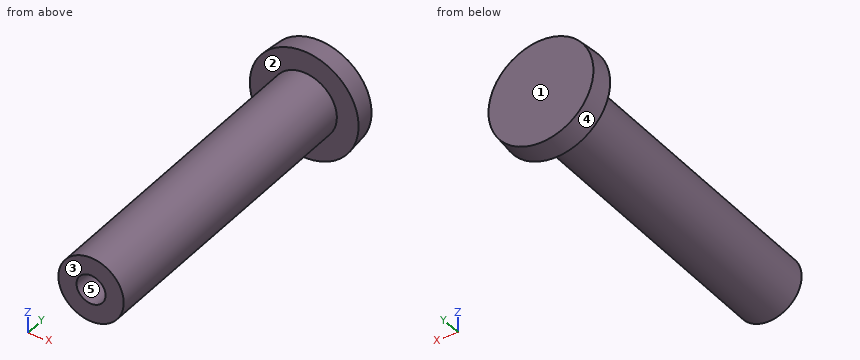
from build123d import *

# Parameters (mm, degrees)
SKETCH1_R           = 2.25
BOSS_EXTRUDE1_DEPTH = 21.5
SKETCH2_R           = 3.75
BOSS_EXTRUDE2_DEPTH = 1.5
BOSS_EXTRUDE2_TAPER = 5
SKETCH3_R           = 1
CUT_EXTRUDE1_DEPTH  = 6
CUT_EXTRUDE1_DRAFT  = -1


with BuildPart() as part:
    # Sketch1 → Boss-Extrude1 (new body)
    with BuildSketch(Plane(origin=(0, 0, 0), x_dir=(1, 0, 0), z_dir=(0, 1, 0))):
        with Locations(Location((0, 0, 0), (0, 0, 270))):
            Circle(SKETCH1_R)
    extrude(amount=BOSS_EXTRUDE1_DEPTH)

    # Sketch2 → Boss-Extrude2 (add)
    with BuildSketch(Plane(origin=(0, 21.5, 0), x_dir=(1, 0, 0), z_dir=(0, 1, 0))):
        Circle(SKETCH2_R)
    extrude(amount=BOSS_EXTRUDE2_DEPTH, taper=BOSS_EXTRUDE2_TAPER)


with BuildPart() as cut_extrude1_tool:
    # Sketch3 → Cut-Extrude1 (with draft: the straight prism first)
    with BuildSketch(Plane.XZ):
        Circle(SKETCH3_R)
    extrude(amount=-CUT_EXTRUDE1_DEPTH)
    # Cut-Extrude1: the draft: its side faces are tilted about the plane it starts from
    cut_extrude1_sides = [cut_extrude1_tool.faces().sort_by_distance(p)[0] for p in [
        (-1, 3, 0),
    ]]
    draft(cut_extrude1_sides, Plane.XZ, CUT_EXTRUDE1_DRAFT)


with BuildPart() as part_1:
    add(part.part)

    # Cut-Extrude1: cut by cut_extrude1_tool
    add(cut_extrude1_tool.part, mode=Mode.SUBTRACT)


solid = part_1.part
Part model, mm, in its own coordinate system. Face numbers are marked on the shaded views. A direction names the side the tool comes from. Coordinates: 2 decimals unless noted, no trailing zeros. Loops run counter-clockwise (first coordinate to the right, second up) from the corner with the lowest first, then second, coordinate; pieces in that order, holes last. Notation, with made-up numbers: (62.5, 24) -> (119.5, 24) arc R27 cw to (119.5, 42) -> close; hole circle Ø8 at (-9, 23). An arc over 180 degrees is marked (long way). Use a Markdown table: item, result. Add a question column.
Item 1: Which spindle directions (+Z, -Z, +X, -X, +Y, -Y) get a long thin tool onto all of the face, cutting with end or side? Do the marked faces 1 and 2. Say none if no direction does.
Item 2: Band-saw the part on A-A on y = 3.25. Write the cut outline in (x, z), plus the area to 3 significant figures.
Item 3: Probe probe 1 along Y at (x, z) = (-1.25, -2); probe 2 along X at (y, z) = (4, -0.25); probe 3 along X at (y, z) = (7.5, 0). List the from-to ranges inside material, lowest first.
Item 4: Pull direction X, two halves, no side cores. Call the marked faces 3, 4 and 5: +X half, -X half, draft (parallel to the pull), parting line (faces both ways), or undercut.
Item 5: Band-saw the part on B-B on y = 15.75. Write the cut outline in (x, z), plus the area to 3 significant figures.
Item 6: Flat gauge pins, fed straight in: P1, Ø0.5, axis at x = 0, z = 0, coming from the -Y side; P2, Ø3, axis at x = 2, y = 12, coming from the -Z side; P3, Ø4, axis at x = -2.5, y = 20.5, coming from the -Z side; P4, Ø1, axis at y = 11.5, z = -3, coming from the +X side. Where does each tip first touch, or does it go through?
Geometry says:
| question | item | result |
|---|---|---|
| 1 | face 1 | +Z, -Z, +X, -X, +Y |
| 1 | face 2 | -Y |
| 2 | outline | circle Ø4.5 at (0, 0); hole circle Ø1.89 at (0, 0) |
| 2 | area | 13.1 mm² |
| 3 | probe 1 | 21.5 to 23 |
| 3 | probe 2 | -2.24 to -0.9, 0.9 to 2.24 |
| 3 | probe 3 | -2.25 to 2.25 |
| 4 | face 3 | draft |
| 4 | face 4 | parting line |
| 4 | face 5 | undercut |
| 5 | outline | circle Ø4.5 at (0, 0) |
| 5 | area | 15.9 mm² |
| 6 | P1 | y = 6 |
| 6 | P2 | z = -2.19 |
| 6 | P3 | z = -3.67 |
| 6 | P4 | through |
